Could you check a few things on this model? Use its own coordinates, in mm. Face numbers are marked on the shaded views. A direction names the side the tool comes from. Give positions to 0.01 mm unless a question says otherwise; leave off trailing zeros. Order: outer loops, then holes, each group sorted by start corner. A loop starts at its lowest first (then second) coordinate and runs counter-clockwise, first axis right, second up. Notation, with made-up numbers: M 26,11.5 L 55,11.5 A14 ccw 55,30.5 Z; hole C 7,-10.5 d6. An arc over 180 degrees is marked long. Use a Markdown table: item, result. Add a question column.
```python
from build123d import *

# Parameters (mm, degrees)
BOSS_EXTRUDE1_DEPTH     = 6
CUT_EXTRUDE1_DEPTH      = 10
CUT_EXTRUDE1_DEPTH_BACK = 2
SKETCH4_R               = 1.05
CUT_EXTRUDE2_DEPTH      = 1.6
SKETCH4_2_R             = 1.05
CUT_EXTRUDE3_DEPTH      = 4


with BuildPart() as part:
    # Sketch1 → Boss-Extrude1 (new body)
    with BuildSketch(Plane(origin=(0, 0, 0), x_dir=(0, 0, -1), z_dir=(1, 0, 0))):
        with BuildLine():
            Line((-11.475, 0), (-5.096628788, 0))
            ThreePointArc((-5.096628788, 0), (-3.969949422, -0.347549212), (-3.234846582, -1.269406393))
            ThreePointArc((-3.234846582, -1.269406393), (3.422206942, -0.603427417), (-2.605598906, 2.299234512))
            ThreePointArc((-2.605598906, 2.299234512), (-3.611663346, 1.6843921), (-4.789264463, 1.743149708))
            Line((-4.789264463, 1.743149708), (-10.782972824, 3.924681145))
            Line((-10.782972824, 3.924681145), (-10.098932537, 5.804066386))
            Line((-10.098932537, 5.804066386), (-5.249850762, 4.039144957))
            ThreePointArc((-5.249850762, 4.039144957), (-4.259008351, 3.942202175), (-3.344188943, 4.334976968))
            ThreePointArc((-3.344188943, 4.334976968), (5.452597189, -0.494781667), (-4.069872513, -3.662207358))
            ThreePointArc((-4.069872513, -3.662207358), (-4.742822691, -3.173037318), (-5.556583933, -3))
            Line((-5.556583933, -3), (-11.475, -3))
            Line((-11.475, -3), (-11.475, -2))
            Line((-11.475, -2), (-11.475, 0))
        make_face()
    extrude(amount=BOSS_EXTRUDE1_DEPTH)

    # Sketch3 → Cut-Extrude1 (cut, two sides: drawn at the far end of the back side and taken through both)
    with BuildSketch(Plane(origin=(0, 1.879385242, -0.684040287), x_dir=(1, 0, 0), z_dir=(0, 0.9396926207859091, -0.34202014332566716)).offset(-CUT_EXTRUDE1_DEPTH_BACK)):
        with BuildLine():
            Line((4.05, -6.550079558), (4.05, -9.550079558))
            ThreePointArc((4.05, -9.550079558), (3, -10.600079558), (1.95, -9.550079558))
            Line((1.95, -9.550079558), (1.95, -6.550079558))
            ThreePointArc((1.95, -6.550079558), (3, -5.500079558), (4.05, -6.550079558))
        make_face()
    extrude(amount=CUT_EXTRUDE1_DEPTH + CUT_EXTRUDE1_DEPTH_BACK, mode=Mode.SUBTRACT)

    # Sketch4 → Cut-Extrude2 (cut)
    with BuildSketch(Plane.XZ.offset(3)):
        Polygon((4.154700538, 10.515791966), (1.845299462, 10.515791966), (0.690598923, 8.515791966), (1.845299462, 6.515791966), (4.154700538, 6.515791966), (5.309401077, 8.515791966), align=None)
        with Locations(Location((3, 8.515791966, 0), (0, 0, 270))):
            Circle(SKETCH4_R, mode=Mode.SUBTRACT)
    extrude(amount=-CUT_EXTRUDE2_DEPTH, mode=Mode.SUBTRACT)

    # Sketch4_2 → Cut-Extrude3 (cut)
    with BuildSketch(Plane.XZ.offset(3)):
        with Locations(Location((3, 8.515791966, 0), (0, 0, 270))):
            Circle(SKETCH4_2_R)
    extrude(amount=-CUT_EXTRUDE3_DEPTH, mode=Mode.SUBTRACT)


solid = part.part
```
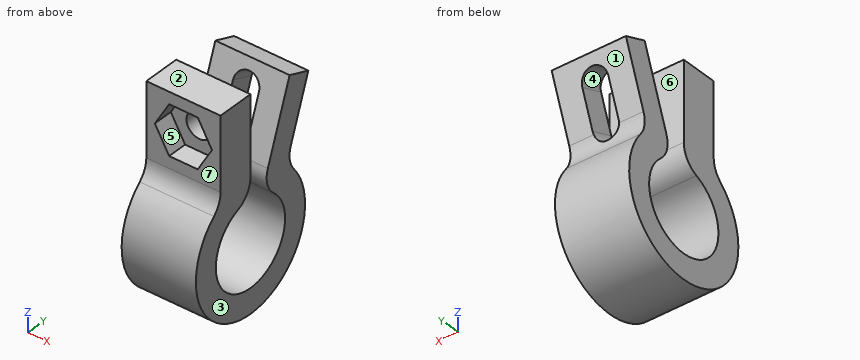
1) Suppose I cut it at C-C on x = 5.5. Please give me the cut outline in (y, z) (3 decimals), and give its area (3 significant figures).
2) For pin 1 (1.3 mm diameter, centred on x = 2.5, y = -2, fed in from -Z); pin 2 (1 mm diameter, centred on x = 1, z = -3.5, fed in from +Y); pin 3 (2.5 mm diameter, centred on x = 3, z = 8.52, fed in from -Y), each with a flat end and sliding along its axis, tell me the tip position at first contact or that it passes through.
3) Suppose I cut it at A-A on z = 0. Please give me the cut outline in (x, y) (3 decimals).
4) Suppose I cut it at D-D on z = -3.75. Please give me the cut outline in (x, y).
5) We'd pull the mould along Z, two halves only. Please class the marked faces 1, 2 and 3: pulls with the +Z half, pulls with the -Z half, needs draft (parallel to the pull), parting line crosses it, or undercut.
6) Suppose I cut it at B-B on x = 3.25. Count the separate pieces of the cut face and the enclosed holes in it, and give its area (3 significant figures).
7) Please list where these lines run through material, in increasing order: line 1 (X direction, y = 3.75, z = 5.75); line 2 (Y direction, x = 4.15, z = 0) (3 decimals); line 3 (Z direction, x = 1.75, y = -2.75) (3 decimals). Write a range as from..to.
8) For the marked faces 4, 5, 6 and 7, which set-ups out of +Z, -Z, +X, -X, +Y, -Y let a thin tool reach every point of the face, with its end or its side?
Values found:
| question | item | result |
|---|---|---|
| 1 | outline | M -3.662,4.07 A5.475 ccw long 4.335,3.344 A2 cw 4.039,5.25 L 5.804,10.099 L 3.925,10.783 L 1.743,4.789 A2 ccw 2.299,2.606 A3.475 cw long -1.269,3.235 A2 ccw 0,5.097 L 0,11.475 L -3,11.475 L -3,5.557 A2 cw Z |
| 1 | area | 83.7 mm^2 |
| 2 | pin 1 | stops at z = -5.31 |
| 2 | pin 2 | stops at y = 4.58 |
| 2 | pin 3 | stops at y = -1.4 |
| 3 | outline | M 0,-5.475 L 6,-5.475 L 6,-3.475 L 0,-3.475 Z; M 0,3.475 L 6,3.475 L 6,5.475 L 0,5.475 Z |
| 4 | outline | M 0,-3.99 L 6,-3.99 L 6,3.99 L 0,3.99 Z |
| 5 | face 1 | undercut |
| 5 | face 2 | pulls with the +Z half |
| 5 | face 3 | needs draft |
| 6 | separate pieces | 3 |
| 6 | enclosed holes | 0 |
| 6 | area | 64.3 mm^2 |
| 7 | line 1 | x = 0..1.95, 4.05..6 |
| 7 | line 2 | y = -5.475..-3.475, 3.475..5.475 |
| 7 | line 3 | z = -4.734..-2.124, 2.124..6.681, 10.351..11.475 |
| 8 | face 4 | none |
| 8 | face 5 | -Y |
| 8 | face 6 | +Z, +X, -X |
| 8 | face 7 | +Z, +X, -X, -Y |
